Autodesk Inventor part; units mm, degrees
ref_plane "YZ Plane" through (0, 0, 0) normal (1, 0, 0) x (0, 1, 0)
ref_plane "XZ Plane" through (0, 0, 0) normal (0, 1, 0) x (-1, 0, 0)
ref_plane "XY Plane" through (0, 0, 0) normal (0, 0, 1) x (1, 0, 0)
sketch "Sketch1" plane through (0, 0, 0) normal (0, 1, 0) x (-1, 0, 0)
  line L0 (-10, -10) -> (10, -10)
  line L1 (10, -10) -> (10, 10)
  line L2 (10, 10) -> (-10, 10)
  line L3 (-10, 10) -> (-10, -10)
  line L4 (-10, -10) -> (10, 10) construction
  line L5 (10, -10) -> (-10, 10) construction
  line L6 (10, 10) -> (30, 10)
  line L7 (30, 10) -> (30, -10)
  line L8 (30, -10) -> (10, -10)
  line L9 (10, -10) -> (10, 10)
  circle A0 centre (30, 10) radius 1.5
  circle A1 centre (30, -10) radius 1.5
  circle A2 centre (10, -10) radius 1.5
  circle A3 centre (10, 10) radius 1.5
  circle A4 centre (-10, 10) radius 1.5
  circle A5 centre (-10, -10) radius 1.5
  line L10 (-15, 22.5) -> (35, 22.5)
  line L11 (35, 22.5) -> (35, -22.5)
  line L12 (35, -22.5) -> (-15, -22.5)
  line L13 (-15, -22.5) -> (-15, 22.5)
  line L14 (-15, 22.5) -> (35, -22.5) construction
  line L15 (35, 22.5) -> (-15, -22.5) construction
  point P0 (0, 0)
  point P1 (10, 0)
  dimension "d0" = 20
  dimension "d1" = 20
  dimension "d2" = 20
  dimension "d3" = 20
  dimension "d4" = 3
  dimension "d5" = 3
  dimension "d6" = 3
  dimension "d7" = 3
  dimension "d8" = 3
  dimension "d9" = 3
  dimension "d10" = 5
  dimension "d11" = 12.5
extrude "Extrusion1" add sketch "Sketch1" along normal blind 4 contours A5 L3 A4 L2 A3 L1 A2 L0 | L1 A3 L6 A0 L7 A1 L8 A2 | L10 L11 L12 L13
fillet "Fillet1" radius 4 1 edges at (15, 0, 0)
sketch "Sketch2" plane through (0, 4, 0) normal (0, 1, 0) x (1, 0, 0)
  line L0 (-35, -22.5) -> (15, -22.5)
  line L1 (15, 22.5) -> (-35, 22.5)
  line L2 (-25, -22.5) -> (6, -22.5)
  line L3 (6, -22.5) -> (6, 22.5)
  line L4 (6, 22.5) -> (-25, 22.5)
  line L5 (-25, 22.5) -> (-25, -22.5)
  line L6 (-35, 22.5) -> (-35, -22.5)
  line L7 (15, -22.5) -> (15, 22.5)
  circle A0 centre (-10, -10) radius 1.5
  circle A1 centre (-10, -10) radius 4.5
  circle A2 centre (-10, 10) radius 1.5
  circle A3 centre (-10, 10) radius 4.5
  point P0 (0, 0)
  point P1 (-6.25, -15)
  point P2 (-13.75, -15)
  point P3 (-13.75, 15)
  point P4 (-6.25, 15)
  dimension "d15" = 10
  dimension "d16" = 9
  dimension "d17" = 9
  dimension "d18" = 9
extrude "Extrusion2" cut sketch "Sketch2" against normal blind 4 contours A0 | A1 | A3
extrude "Extrusion3" add sketch "Sketch2" along normal blind 160 contours L5 L1 L3 L0 | A0 | A1 | A2 | A3
fillet "Fillet2" radius 8 2 edges at (-35, 2, 22.5) (-35, 2, -22.5)
sketch "Sketch3" plane through (-25, 164, 22.5) normal (0, 0, 1) x (1, 0, 0)
  line L0 (31, 0) -> (0, 0)
  circle A0 centre (15.8021, -15) radius 10
  circle A1 centre (15.8021, -5) radius 1
  circle A2 centre (19.2223, -5.6031) radius 1
  circle A3 centre (22.8732, -7.9289) radius 1
  line L1 (15.8021, -15) -> (19.2223, -5.6031)
  line L2 (15.8021, -15) -> (22.8732, -7.9289)
  circle A4 centre (5.8021, -15) radius 1
  circle A5 centre (15.8021, -25) radius 1
  circle A6 centre (25.8021, -15) radius 1
  circle A7 centre (6.4052, -11.5798) radius 1
  circle A8 centre (12.3819, -24.3969) radius 1
  circle A9 centre (25.199, -18.4202) radius 1
  circle A10 centre (8.731, -7.9289) radius 1
  circle A11 centre (8.731, -22.0711) radius 1
  circle A12 centre (22.8732, -22.0711) radius 1
  line L3 (15.8021, -15) -> (15.8021, 0)
  point P0 (25, -164)
  dimension "d24" = 20
  dimension "d26" = 2
  dimension "d27" = 2
  dimension "d30" = 2
  dimension "d33" = 360
  dimension "d37" = 360
  dimension "d41" = 360
  dimension "d54" = 15
  dimension "d55" = 45
  dimension "d56" = 20
extrude "Extrusion4" cut sketch "Sketch3" against normal blind 100 contours A0 A6 | A0 A6 | A3 L2 A0 | A0 A3 | A9 A0 | A0 A9 | L2 A3 A0 | A12 A0 | A0 A12 | A2 L1 A0 | A0 A2 | A2 A0 L1 | L3 A0 A1 | A1 A0 L3 | A1 L3 A0 | A0 L3 A1 | A5 A0 | A0 A5 | A10 A0 | A0 A10 | A8 A0 | A0 A8 | A7 A0 | A0 A7 | A11 A0 | A0 A11 | A4 A0 | A0 A4
sketch "Sketch4" plane through (0, 164, 0) normal (0, 1, 0) x (1, 0, 0)
  line L0 (-25, 22.5) -> (-25, -22.5)
  line L1 (6, 22.5) -> (-25, 22.5)
  line L2 (-25, -12.5) -> (6, -12.5)
  line L3 (6, -12.5) -> (6, 22.5)
  line L4 (6, 22.5) -> (-25, 22.5)
  line L5 (-25, 22.5) -> (-25, -12.5)
  line L6 (-25, -22.5) -> (6, -22.5)
  point P0 (0, 0)
  dimension "d45" = 10
extrude "Extrusion5" cut sketch "Sketch4" against normal blind 140
fillet "Fillet3" radius 8 1 edges at (-9.5, 24, 12.5)
fillet "Fillet4" radius 8 2 edges at (-25, 164, 17.5) (6, 164, 17.5)
fillet "Fillet5" radius 8 1 edges at (-9.5, 24, -22.5)
sketch "Sketch5" plane through (6, 4, 22.5) normal (1, 0, 0) x (0, 0, -1)
  line L0 (10, 28) -> (10, 152)
  line L1 (18, 20) -> (37, 20)
  line L2 (10, 99.4385) -> (37, 20)
  arc A0 (45, 12) -> (37, 20) centre (37, 12) ccw
  line L3 (10, 114.9758) -> (45, 12)
  arc A1 (45, 12) -> (37, 20) centre (37, 12) ccw
  line L4 (37, 20) -> (18, 20)
  arc A2 (10, 28) -> (18, 20) centre (18, 28) ccw
  line L5 (10, 28) -> (10, 152)
  line L6 (0, 152) -> (10, 152)
  line L7 (0, 0) -> (0, 152)
  line L8 (45, 0) -> (0, 0)
  line L9 (45, 0) -> (45, 12)
  point P0 (22.5, -4)
  point P1 (43.3431, 16.875)
  dimension "d51" = 5
extrude "Extrusion6" add sketch "Sketch5" against normal up to surface (31 mm away) contours L0 L3 A0 L2
sketch "Sketch6" plane through (6, 4, 22.5) normal (0, 0, 1) x (1, 0, 0)
  circle A0 centre (-15.1979, 155) radius 1
  circle A1 centre (-15.1979, 135) radius 1
  line L0 (-15.1979, 155) -> (-15.1979, 135)
  circle A2 centre (-15.1979, 145) radius 1.5
  point P0 (-6, -4)
  dimension "d57" = 3
extrude "Extrusion7" cut sketch "Sketch6" against normal blind 20 contours A2 L0 | L0 A2
properties part number "Vertical_Stereo_1"
Design review of the part built by this model. Coordinates are the model's own, in mm. A direction names the side the tool comes from. Round coordinates to 2 decimals unless told otherwise and drop trailing zeros. Write each loop counter-clockwise with the first axis right and the second up, starting at its lowest first coordinate (ties: lowest second). Pieces come first, ordered by that corner, then holes. Notation, with made-up numbers: (-30, 38.25) -> (-25, 38.25) arc R22 ccw to (-25, 55.25) -> close; hole circle Ø4 at (64.25, 17.25). An arc over 180 degrees is marked (long way). Write item = value, one per line. Start each with the question number.
1) Wall thickness on probe 1 along Z at (x, y) = (10, 2); probe 2 along Z at (x, y) = (-10, 2.7); probe 3 along X at (y, z) = (149, 18): over which ranges is each line inside the solid? List them lowest first. Write a range as from..to.
2) Take a section at B-B, the plane x = -30. State the section outline as (y, z) points, plus the area to 3 significant figures.
3) Take a section at C-C, the plane x = -22. State the section outline as (y, z) points (1 decimal), plus the area to 3 significant figures.
4) Tool access review of faces 4 (the face through (-9.28, 64.28, -0.81)), 5 (the face through (-10, 4, -10)), 6 (the face through (11, 4, 0)): name each direction out of +Z, -Z, +X, -X, +Y, -Y from which nothing blocks a thin tool from reaching the whole face with its end or side.
5) Take a section at D-D, the plane y = 10. State the section outline as (x, z) points.
6) Clearance check with flat-ended pins moving along their axes: pin 1 (25 mm diameter, centred on x = -12.5, y = 55, fed in from -Z); pin 2 (5 mm diameter, centred on x = -31, z = -3.5, fed in from +Y); pin 3 (13.5 mm diameter, centred on y = 115, z = 7.5, fed in from +X); pin 4 (1 mm diameter, centred on y = 98.5, z = 4, fed in from -X). State where each tip first meets the part, or that it passes through.
7) Mouldability with a two-part tool opening along X and no side actions: class faces 1 (the face through (-32.719, 2.028, 20.094)), 2 (the face through (-5.708, 2.028, -11.352)), 3 (the face through (6, 64, 15)) as +X half, -X half, draft (parallel to the pull), parting line (faces both ways), or undercut.
Results list:
q1.probe_1 = -22.5..-11.5, -8.5..8.5, 11.5..22.5
q1.probe_2 = -22.5..-14.5, -5.5..5.5, 14.5..22.5
q1.probe_3 = -25..-20.2, -18.2..-10.7, -7.7..-0.2, 1.8..6
q2.outline = (0, -21.92) -> (4, -21.92) -> (4, -11.5) -> (0, -11.5) -> close; (0, -8.5) -> (4, -8.5) -> (4, 8.5) -> (0, 8.5) -> close; (0, 11.5) -> (4, 11.5) -> (4, 21.92) -> (0, 21.92) -> close
q2.area = 151 mm²
q3.outline = (0, -22.5) -> (16, -22.5) arc R8 ccw to (20.9, -20.8) -> (119, 12.5) -> (162.2, 12.5) -> (162.2, 22.5) -> (0, 22.5) -> close; hole (24, -14.5) -> (103.4, 12.5) -> (32, 12.5) arc R8 ccw to (24, 4.5) -> close
q3.area = 2,930 mm²
q4.face_4 = +X, -X
q4.face_5 = -Y
q4.face_6 = +Z, -Z, +X, +Y
q5.outline = (-25, -22.5) -> (6, -22.5) -> (6, 22.5) -> (-25, 22.5) -> close
q6.pin_1 = -13.49
q6.pin_2 = 4
q6.pin_3 = 6
q6.pin_4 = through
q7.face_1 = -X half
q7.face_2 = undercut
q7.face_3 = +X half
